```python
from build123d import *


with BuildPart() as f1:
    # F0 (on Front) → F1 (revolve)
    with BuildSketch(Plane.XZ):
        with BuildLine():
            Line((20.5, 50), (0, 50))
            Line((0, 50), (0, 0))
            Line((0, 0), (45, 0))
            Line((45, 0), (45, 15))
            ThreePointArc((45, 15), (43.535534, 18.535534), (40, 20))
            Line((40, 20), (38.333333, 20))
            ThreePointArc((38.333333, 20), (35.559832, 20.839749), (33.717949, 23.076923))
            Line((33.717949, 23.076923), (23.269231, 48.153846))
            ThreePointArc((23.269231, 48.153846), (22.164101, 49.496151), (20.5, 50))
        make_face()
    revolve(axis=Axis((0, 0, 11.951942), (0, 0, -1)))


solid = f1.part
```
Input: part model. Units: mm. Frame: model coordinates. Round coordinates to 2 decimals unless told otherwise and drop trailing zeros. Write each loop counter-clockwise with the first axis right and the second up, starting at its lowest first coordinate (ties: lowest second). Pieces come first, ordered by that corner, then holes. Notation, with made-up numbers: (63.5, 38) - (99.5, 38) arc R26 ccw to (99.5, 67) - close; hole circle Ø6 at (44.5, 42.25). An arc over 180 degrees is marked (long way). Write item = value, one per line.
(1) Contact query for flat-ended pins moving along their axis: pin 1 Ø1.5 at (y, z) = (-16.5, 10) entering from -X; pin 2 Ø2 at (y, z) = (16.5, 6.5) entering from +X; pin 3 Ø12 at (y, z) = (-25.5, 19) entering from -X. Output: stop coordinate, or through.
Geometry check:
pin_1 = -42.15
pin_2 = 42.25
pin_3 = -40.05
(2) Pull-direction query (X, two-part tool) for faces 1 (the flat face through (0, 0, 50)), 2 (the cylindrical face through (20.765, 39.923, 7.605)); classes: +X half, -X half, draft (parallel to the pull), parting line (faces both ways), or undercut.
Geometry check:
face_1 = draft
face_2 = parting line
(3) Section query D-D on z = 33.5. Output: boundary loops of the cut face in (x, y) (3 decimals), then the cut area to 3 significant figures.
Geometry check:
outline = circle Ø58.75 at (0, 0)
area = 2,710 mm^2
(4) Material intervals for probe 1 along Z at (x, y) = (-3.5, 39.5); probe 2 along X at (y, z) = (-1.5, 36.5); probe 3 along Y at (x, z) = (-9.5, 47), sorted ascending.
Geometry check:
probe_1 = 0 to 20
probe_2 = -28.08 to 28.08
probe_3 = -21.77 to 21.77
(5) Section query C-C on z = 44.5. Output: boundary loops of the cut face in (x, y).
Geometry check:
outline = circle Ø49.58 at (0, 0)
(6) Section query A-A on x = 0. Output: boundary loops of the cut face in (y, z).
Geometry check:
outline = (-45, 0) - (45, 0) - (45, 15) arc R5 ccw to (40, 20) - (38.33, 20) arc R5 cw to (33.72, 23.08) - (23.27, 48.15) arc R3 ccw to (20.5, 50) - (-20.5, 50) arc R3 ccw to (-23.27, 48.15) - (-33.72, 23.08) arc R5 cw to (-38.33, 20) - (-40, 20) arc R5 ccw to (-45, 15) - close
